```python
from build123d import *

# Parameters (mm, degrees)
F0_W     = 370
F0_H     = 390
F1_DEPTH = 5
F2_D     = 5.5
F2_DEPTH = 17
F3_D     = 6.5
F3_DEPTH = 17
F4_SIZE  = 5


with BuildPart() as f1:
    # F0 (on Top) → F1 (new body)
    with BuildSketch(Plane.XY):
        with Locations((0, -10)):
            Rectangle(F0_W, F0_H)
        with BuildLine():
            ThreePointArc((-140, 120), (-134.142136, 134.142136), (-120, 140))
            Line((-120, 140), (120, 140))
            ThreePointArc((120, 140), (134.142136, 134.142136), (140, 120))
            Line((140, 120), (140, -120))
            ThreePointArc((140, -120), (134.142136, -134.142136), (120, -140))
            Line((120, -140), (-120, -140))
            ThreePointArc((-120, -140), (-134.142136, -134.142136), (-140, -120))
            Line((-140, -120), (-140, 120))
        make_face(mode=Mode.SUBTRACT)
    extrude(amount=-F1_DEPTH)

    # F2
    with Locations(Plane.XY):
        with Locations((-175, 87.5), (-175, 0), (-175, -87.5), (-87.5, -175), (0, -175), (87.5, -175), (175, -87.5), (175, 87.5), (87.5, 175), (0, 175), (-87.5, 175), (175, 0)):
            Hole(F2_D / 2, depth=F2_DEPTH)

    # F3
    with Locations(Plane.XY):
        with Locations((-175, -175), (-175, 175), (175, 175), (175, -175)):
            Hole(F3_D / 2, depth=F3_DEPTH)

    # F4
    f4_edges = [f1.edges().sort_by_distance(p)[0] for p in [
        (-185, -205, -2.5),
        (185, -205, -2.5),
        (185, 185, -2.5),
        (-185, 185, -2.5),
    ]]
    chamfer(f4_edges, length=F4_SIZE)


solid = f1.part
```
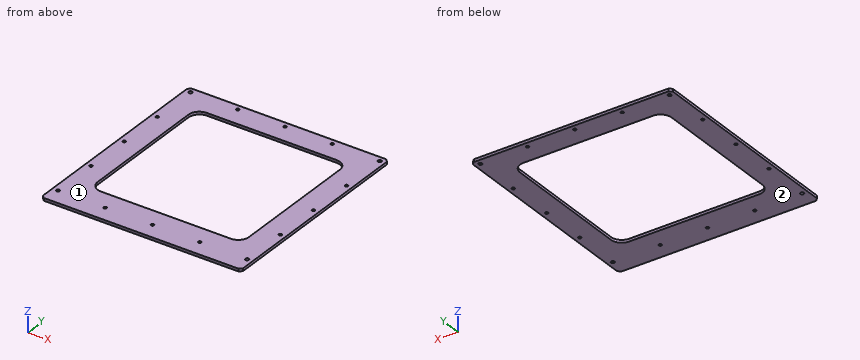
Geometry check sheet. Reference: the model listing, model coordinates, mm. Face numbers are marked on the shaded views. Coordinates: 2 decimals unless noted, no trailing zeros. Order: outer loops, then holes, each group sorted by start corner. A loop starts at its lowest first (then second) coordinate and runs counter-clockwise, first axis right, second up.
Item 1: Section check A-A (z = -3.55). Count the separate pieces of the cut face and the enclosed holes in it, plus the area to 3 significant figures.
Item 2: Section check C-C (x = 34.5). Enter the section's corners in (y, z), plus the area to 3 significant figures.
Item 3: Scan lines: line 1 along Y through (x, z) = (-175, -3.5); line 2 along X through (y, z) = (-175, -3.45); line 3 along Y through (x, z) = (0, -3.9). Record each from-to range of solid material in increasing order.
Item 4: Mould release check, pull along Z, two halves, no side actions. Record for the marked faces 1 and 2: released by +Z, released by -Z, zero draft, split by the parting line, or undercut.
Item 5: Section check B-B (y = -17.5). Enter the section's corners in (x, z).
Check sheet entries:
1. separate pieces: 1
1. enclosed holes: 17
1. area: 65,800 mm2
2. outline: (-205, -5) - (-140, -5) - (-140, 0) - (-205, 0) - close; (140, -5) - (185, -5) - (185, 0) - (140, 0) - close
2. area: 550 mm2
3. line 1: y = -205 to -178.25, -171.75 to -90.25, -84.75 to -2.75, 2.75 to 84.75, 90.25 to 171.75, 178.25 to 185
3. line 2: x = -185 to -178.25, -171.75 to -90.25, -84.75 to -2.75, 2.75 to 84.75, 90.25 to 171.75, 178.25 to 185
3. line 3: y = -205 to -177.75, -172.25 to -140, 140 to 172.25, 177.75 to 185
4. face 1: released by +Z
4. face 2: released by -Z
5. outline: (-185, -5) - (-140, -5) - (-140, 0) - (-185, 0) - close; (140, -5) - (185, -5) - (185, 0) - (140, 0) - close
